Source: CAD feature listing. Evaluate the final solid. Frame: model axes, mm. Round coordinates to 2 decimals unless told otherwise and drop trailing zeros. Loops run counter-clockwise (first coordinate to the right, second up) from the corner with the lowest first, then second, coordinate; pieces in that order, holes last.
Item 1: Section query B-B on x = 1.55. Give the number of separate pieces and of enclosed holes in the cut face, then the cut area to 4 significant figures.
Item 2: Section query A-A on y = 10. Return loops of the section in (x, z).
Item 3: Section query D-D on y = 0.5. Return loops of the section in (x, z), then the cut area to 3 significant figures.
Item 4: Ray query, L1, parallel to Z at x = -1.75, y = 1; L2, parallel to X at y = 11.5, z = -0.4; L3, parallel to Z at x = -1.65, y = 5. Return the intervals inside material, ascending.
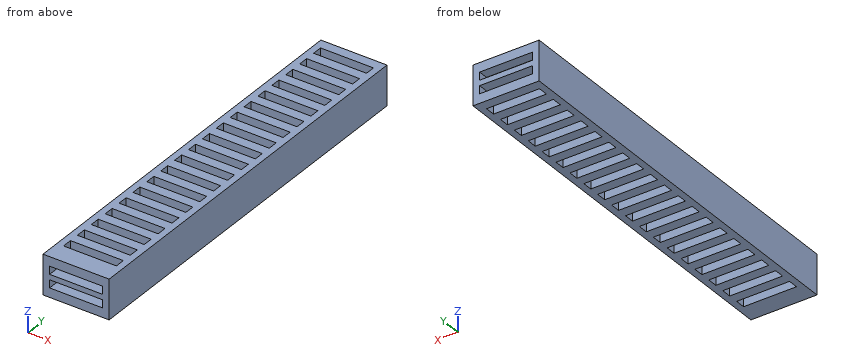
```python
from build123d import *

# Parameters (mm, degrees)
SKETCH1_W                = 5
SKETCH1_H                = 3
BOSS_EXTRUDE1_DEPTH      = 15
CUT_EXTRUDE1_START       = -31
SKETCH2_W                = 4
SKETCH2_H                = 0.6
CUT_EXTRUDE1_DEPTH       = 32
SKETCH3_W                = 4
SKETCH3_H                = 0.75
CUT_EXTRUDE2_DEPTH       = 0.7
LPATTERN1_COUNT          = 19
LPATTERN1_PITCH          = 1.5
MIRROR2_COPY_1_SKETCH_W  = 4
MIRROR2_COPY_1_SKETCH_H  = 0.75
MIRROR2_COPY_1_DEPTH     = 0.7
MIRROR2_COPY_2_SKETCH_W  = 4
MIRROR2_COPY_2_SKETCH_H  = 0.75
MIRROR2_COPY_2_DEPTH     = 0.7
MIRROR2_COPY_3_SKETCH_W  = 4
MIRROR2_COPY_3_SKETCH_H  = 0.75
MIRROR2_COPY_3_DEPTH     = 0.7
MIRROR2_COPY_4_SKETCH_W  = 4
MIRROR2_COPY_4_SKETCH_H  = 0.75
MIRROR2_COPY_4_DEPTH     = 0.7
MIRROR2_COPY_5_SKETCH_W  = 4
MIRROR2_COPY_5_SKETCH_H  = 0.75
MIRROR2_COPY_5_DEPTH     = 0.7
MIRROR2_COPY_6_SKETCH_W  = 4
MIRROR2_COPY_6_SKETCH_H  = 0.75
MIRROR2_COPY_6_DEPTH     = 0.7
MIRROR2_COPY_7_SKETCH_W  = 4
MIRROR2_COPY_7_SKETCH_H  = 0.75
MIRROR2_COPY_7_DEPTH     = 0.7
MIRROR2_COPY_8_SKETCH_W  = 4
MIRROR2_COPY_8_SKETCH_H  = 0.75
MIRROR2_COPY_8_DEPTH     = 0.7
MIRROR2_COPY_9_SKETCH_W  = 4
MIRROR2_COPY_9_SKETCH_H  = 0.75
MIRROR2_COPY_9_DEPTH     = 0.7
MIRROR2_COPY_10_SKETCH_W = 4
MIRROR2_COPY_10_SKETCH_H = 0.75
MIRROR2_COPY_10_DEPTH    = 0.7
MIRROR2_COPY_11_SKETCH_W = 4
MIRROR2_COPY_11_SKETCH_H = 0.75
MIRROR2_COPY_11_DEPTH    = 0.7
MIRROR2_COPY_12_SKETCH_W = 4
MIRROR2_COPY_12_SKETCH_H = 0.75
MIRROR2_COPY_12_DEPTH    = 0.7
MIRROR2_COPY_13_SKETCH_W = 4
MIRROR2_COPY_13_SKETCH_H = 0.75
MIRROR2_COPY_13_DEPTH    = 0.7
MIRROR2_COPY_14_SKETCH_W = 4
MIRROR2_COPY_14_SKETCH_H = 0.75
MIRROR2_COPY_14_DEPTH    = 0.7
MIRROR2_COPY_15_SKETCH_W = 4
MIRROR2_COPY_15_SKETCH_H = 0.75
MIRROR2_COPY_15_DEPTH    = 0.7
MIRROR2_COPY_16_SKETCH_W = 4
MIRROR2_COPY_16_SKETCH_H = 0.75
MIRROR2_COPY_16_DEPTH    = 0.7
MIRROR2_COPY_17_SKETCH_W = 4
MIRROR2_COPY_17_SKETCH_H = 0.75
MIRROR2_COPY_17_DEPTH    = 0.7
MIRROR2_COPY_18_SKETCH_W = 4
MIRROR2_COPY_18_SKETCH_H = 0.75
MIRROR2_COPY_18_DEPTH    = 0.7


with BuildPart() as part:
    # Sketch1 → Boss-Extrude1 (new body, symmetric)
    with BuildSketch(Plane(origin=(0, 0, 0), x_dir=(1, 0, 0), z_dir=(0, 1, 0))):
        Rectangle(SKETCH1_W, SKETCH1_H)
    extrude(amount=BOSS_EXTRUDE1_DEPTH, both=True)

    # Sketch2 → Cut-Extrude1 (cut)
    with BuildSketch(Plane(origin=(0, 15, 0), x_dir=(1, 0, 0), z_dir=(0, 1, 0)).offset(CUT_EXTRUDE1_START)):
        with Locations((0, 0.5)):
            Rectangle(SKETCH2_W, SKETCH2_H)
    cut_extrude1 = extrude(amount=CUT_EXTRUDE1_DEPTH, mode=Mode.SUBTRACT)

    # Mirror1: Cut-Extrude1 across plane
    add(cut_extrude1.mirror(Plane.XY), mode=Mode.SUBTRACT)

    # Sketch3 → Cut-Extrude2 (cut)
    with BuildSketch(Plane.XY.offset(1.5)):
        with Locations((0, 13.875)):
            Rectangle(SKETCH3_W, SKETCH3_H)
    cut_extrude2 = extrude(amount=-CUT_EXTRUDE2_DEPTH, mode=Mode.SUBTRACT)

    # LPattern1: Cut-Extrude2 ×19
    with Locations(*[(0, -i * LPATTERN1_PITCH, 0) for i in range(1, LPATTERN1_COUNT)]):
        add(cut_extrude2, mode=Mode.SUBTRACT)

    # Mirror2: Cut-Extrude2 across plane
    add(cut_extrude2.mirror(Plane.XY), mode=Mode.SUBTRACT)

    # Mirror2 copy 1 sketch → Mirror2 copy 1 (cut)
    with BuildSketch(Plane(origin=(0, -1.5, -1.5), x_dir=(1, 0, 0), z_dir=(0, 0, -1))):
        with Locations((0, -13.875)):
            Rectangle(MIRROR2_COPY_1_SKETCH_W, MIRROR2_COPY_1_SKETCH_H)
    extrude(amount=-MIRROR2_COPY_1_DEPTH, mode=Mode.SUBTRACT)

    # Mirror2 copy 2 sketch → Mirror2 copy 2 (cut)
    with BuildSketch(Plane(origin=(0, -3, -1.5), x_dir=(1, 0, 0), z_dir=(0, 0, -1))):
        with Locations((0, -13.875)):
            Rectangle(MIRROR2_COPY_2_SKETCH_W, MIRROR2_COPY_2_SKETCH_H)
    extrude(amount=-MIRROR2_COPY_2_DEPTH, mode=Mode.SUBTRACT)

    # Mirror2 copy 3 sketch → Mirror2 copy 3 (cut)
    with BuildSketch(Plane(origin=(0, -4.5, -1.5), x_dir=(1, 0, 0), z_dir=(0, 0, -1))):
        with Locations((0, -13.875)):
            Rectangle(MIRROR2_COPY_3_SKETCH_W, MIRROR2_COPY_3_SKETCH_H)
    extrude(amount=-MIRROR2_COPY_3_DEPTH, mode=Mode.SUBTRACT)

    # Mirror2 copy 4 sketch → Mirror2 copy 4 (cut)
    with BuildSketch(Plane(origin=(0, -6, -1.5), x_dir=(1, 0, 0), z_dir=(0, 0, -1))):
        with Locations((0, -13.875)):
            Rectangle(MIRROR2_COPY_4_SKETCH_W, MIRROR2_COPY_4_SKETCH_H)
    extrude(amount=-MIRROR2_COPY_4_DEPTH, mode=Mode.SUBTRACT)

    # Mirror2 copy 5 sketch → Mirror2 copy 5 (cut)
    with BuildSketch(Plane(origin=(0, -7.5, -1.5), x_dir=(1, 0, 0), z_dir=(0, 0, -1))):
        with Locations((0, -13.875)):
            Rectangle(MIRROR2_COPY_5_SKETCH_W, MIRROR2_COPY_5_SKETCH_H)
    extrude(amount=-MIRROR2_COPY_5_DEPTH, mode=Mode.SUBTRACT)

    # Mirror2 copy 6 sketch → Mirror2 copy 6 (cut)
    with BuildSketch(Plane(origin=(0, -9, -1.5), x_dir=(1, 0, 0), z_dir=(0, 0, -1))):
        with Locations((0, -13.875)):
            Rectangle(MIRROR2_COPY_6_SKETCH_W, MIRROR2_COPY_6_SKETCH_H)
    extrude(amount=-MIRROR2_COPY_6_DEPTH, mode=Mode.SUBTRACT)

    # Mirror2 copy 7 sketch → Mirror2 copy 7 (cut)
    with BuildSketch(Plane(origin=(0, -10.5, -1.5), x_dir=(1, 0, 0), z_dir=(0, 0, -1))):
        with Locations((0, -13.875)):
            Rectangle(MIRROR2_COPY_7_SKETCH_W, MIRROR2_COPY_7_SKETCH_H)
    extrude(amount=-MIRROR2_COPY_7_DEPTH, mode=Mode.SUBTRACT)

    # Mirror2 copy 8 sketch → Mirror2 copy 8 (cut)
    with BuildSketch(Plane(origin=(0, -12, -1.5), x_dir=(1, 0, 0), z_dir=(0, 0, -1))):
        with Locations((0, -13.875)):
            Rectangle(MIRROR2_COPY_8_SKETCH_W, MIRROR2_COPY_8_SKETCH_H)
    extrude(amount=-MIRROR2_COPY_8_DEPTH, mode=Mode.SUBTRACT)

    # Mirror2 copy 9 sketch → Mirror2 copy 9 (cut)
    with BuildSketch(Plane(origin=(0, -13.5, -1.5), x_dir=(1, 0, 0), z_dir=(0, 0, -1))):
        with Locations((0, -13.875)):
            Rectangle(MIRROR2_COPY_9_SKETCH_W, MIRROR2_COPY_9_SKETCH_H)
    extrude(amount=-MIRROR2_COPY_9_DEPTH, mode=Mode.SUBTRACT)

    # Mirror2 copy 10 sketch → Mirror2 copy 10 (cut)
    with BuildSketch(Plane(origin=(0, -15, -1.5), x_dir=(1, 0, 0), z_dir=(0, 0, -1))):
        with Locations((0, -13.875)):
            Rectangle(MIRROR2_COPY_10_SKETCH_W, MIRROR2_COPY_10_SKETCH_H)
    extrude(amount=-MIRROR2_COPY_10_DEPTH, mode=Mode.SUBTRACT)

    # Mirror2 copy 11 sketch → Mirror2 copy 11 (cut)
    with BuildSketch(Plane(origin=(0, -16.5, -1.5), x_dir=(1, 0, 0), z_dir=(0, 0, -1))):
        with Locations((0, -13.875)):
            Rectangle(MIRROR2_COPY_11_SKETCH_W, MIRROR2_COPY_11_SKETCH_H)
    extrude(amount=-MIRROR2_COPY_11_DEPTH, mode=Mode.SUBTRACT)

    # Mirror2 copy 12 sketch → Mirror2 copy 12 (cut)
    with BuildSketch(Plane(origin=(0, -18, -1.5), x_dir=(1, 0, 0), z_dir=(0, 0, -1))):
        with Locations((0, -13.875)):
            Rectangle(MIRROR2_COPY_12_SKETCH_W, MIRROR2_COPY_12_SKETCH_H)
    extrude(amount=-MIRROR2_COPY_12_DEPTH, mode=Mode.SUBTRACT)

    # Mirror2 copy 13 sketch → Mirror2 copy 13 (cut)
    with BuildSketch(Plane(origin=(0, -19.5, -1.5), x_dir=(1, 0, 0), z_dir=(0, 0, -1))):
        with Locations((0, -13.875)):
            Rectangle(MIRROR2_COPY_13_SKETCH_W, MIRROR2_COPY_13_SKETCH_H)
    extrude(amount=-MIRROR2_COPY_13_DEPTH, mode=Mode.SUBTRACT)

    # Mirror2 copy 14 sketch → Mirror2 copy 14 (cut)
    with BuildSketch(Plane(origin=(0, -21, -1.5), x_dir=(1, 0, 0), z_dir=(0, 0, -1))):
        with Locations((0, -13.875)):
            Rectangle(MIRROR2_COPY_14_SKETCH_W, MIRROR2_COPY_14_SKETCH_H)
    extrude(amount=-MIRROR2_COPY_14_DEPTH, mode=Mode.SUBTRACT)

    # Mirror2 copy 15 sketch → Mirror2 copy 15 (cut)
    with BuildSketch(Plane(origin=(0, -22.5, -1.5), x_dir=(1, 0, 0), z_dir=(0, 0, -1))):
        with Locations((0, -13.875)):
            Rectangle(MIRROR2_COPY_15_SKETCH_W, MIRROR2_COPY_15_SKETCH_H)
    extrude(amount=-MIRROR2_COPY_15_DEPTH, mode=Mode.SUBTRACT)

    # Mirror2 copy 16 sketch → Mirror2 copy 16 (cut)
    with BuildSketch(Plane(origin=(0, -24, -1.5), x_dir=(1, 0, 0), z_dir=(0, 0, -1))):
        with Locations((0, -13.875)):
            Rectangle(MIRROR2_COPY_16_SKETCH_W, MIRROR2_COPY_16_SKETCH_H)
    extrude(amount=-MIRROR2_COPY_16_DEPTH, mode=Mode.SUBTRACT)

    # Mirror2 copy 17 sketch → Mirror2 copy 17 (cut)
    with BuildSketch(Plane(origin=(0, -25.5, -1.5), x_dir=(1, 0, 0), z_dir=(0, 0, -1))):
        with Locations((0, -13.875)):
            Rectangle(MIRROR2_COPY_17_SKETCH_W, MIRROR2_COPY_17_SKETCH_H)
    extrude(amount=-MIRROR2_COPY_17_DEPTH, mode=Mode.SUBTRACT)

    # Mirror2 copy 18 sketch → Mirror2 copy 18 (cut)
    with BuildSketch(Plane(origin=(0, -27, -1.5), x_dir=(1, 0, 0), z_dir=(0, 0, -1))):
        with Locations((0, -13.875)):
            Rectangle(MIRROR2_COPY_18_SKETCH_W, MIRROR2_COPY_18_SKETCH_H)
    extrude(amount=-MIRROR2_COPY_18_DEPTH, mode=Mode.SUBTRACT)


solid = part.part
```
Data:
1. separate pieces: 41
1. enclosed holes: 0
1. area: 34.05 mm2
2. outline: (-2.5, -1.5) - (2.5, -1.5) - (2.5, 1.5) - (-2.5, 1.5) - close; hole (-2, -0.8) - (2, -0.8) - (2, -0.2) - (-2, -0.2) - close; hole (-2, 0.2) - (2, 0.2) - (2, 0.8) - (-2, 0.8) - close
3. outline: (-2.5, -1.5) - (-2, -1.5) - (-2, -0.2) - (2, -0.2) - (2, -1.5) - (2.5, -1.5) - (2.5, 1.5) - (2, 1.5) - (2, 0.2) - (-2, 0.2) - (-2, 1.5) - (-2.5, 1.5) - close
3. area: 4.60 mm2
4. L1: z = -1.5 to -0.8, -0.2 to 0.2, 0.8 to 1.5
4. L2: x = -2.5 to -2, 2 to 2.5
4. L3: z = -0.2 to 0.2
